from build123d import *

# Parameters (mm, degrees)
SKETCH1_R           = 7.5
SKETCH1_R_2         = 15
SKETCH1_R_3         = 11
SKETCH1_R_4         = 5
BOSS_EXTRUDE1_DEPTH = 10
SKETCH1_5_R         = 7.5
SKETCH1_5_R_2       = 5
BOSS_EXTRUDE2_DEPTH = 40
SKETCH2_R           = 7.5
SKETCH2_R_2         = 15
BOSS_EXTRUDE5_DEPTH = 10
SKETCH2_6_R         = 7.5
SKETCH2_6_R_2       = 5
BOSS_EXTRUDE6_DEPTH = 15
SKETCH2_7_R         = 15
SKETCH2_7_R_2       = 11
BOSS_EXTRUDE7_DEPTH = 30


with BuildPart() as part:
    # Sketch1 → Boss-Extrude1 (new body)
    # profile 1 of 6: a face of its own
    with BuildSketch(Plane(origin=(0, 0, 0), x_dir=(1, 0, 0), z_dir=(0, 1, 0))):
        with BuildLine():
            Line((-25, 35), (25, 35))
            ThreePointArc((25, 35), (32.071067812, 32.071067812), (35, 25))
            Line((35, 25), (35, -25))
            ThreePointArc((35, -25), (32.071067812, -32.071067812), (25, -35))
            Line((25, -35), (-25, -35))
            ThreePointArc((-25, -35), (-32.071067812, -32.071067812), (-35, -25))
            Line((-35, -25), (-35, 25))
            ThreePointArc((-35, 25), (-32.071067812, 32.071067812), (-25, 35))
        make_face()
        with Locations((25, -25)):
            Circle(SKETCH1_R, mode=Mode.SUBTRACT)
        Circle(SKETCH1_R_2, mode=Mode.SUBTRACT)
        with Locations((-25, 25)):
            Circle(SKETCH1_R, mode=Mode.SUBTRACT)
        with Locations((25, 25)):
            Circle(SKETCH1_R, mode=Mode.SUBTRACT)
        with Locations((-25, -25)):
            Circle(SKETCH1_R, mode=Mode.SUBTRACT)
    # profile 2 of 6: a face of its own
    with BuildSketch(Plane(origin=(0, 0, 0), x_dir=(1, 0, 0), z_dir=(0, 1, 0))):
        Circle(SKETCH1_R_2)
        with Locations(Location((0, 0, 0), (0, 0, 270))):
            Circle(SKETCH1_R_3, mode=Mode.SUBTRACT)
    # profile 3 of 6: a face of its own
    with BuildSketch(Plane(origin=(0, 0, 0), x_dir=(1, 0, 0), z_dir=(0, 1, 0))):
        with Locations((-25, -25)):
            Circle(SKETCH1_R)
        with Locations(Location((-25, -25, 0), (0, 0, 270))):
            Circle(SKETCH1_R_4, mode=Mode.SUBTRACT)
    # profile 4 of 6: a face of its own
    with BuildSketch(Plane(origin=(0, 0, 0), x_dir=(1, 0, 0), z_dir=(0, 1, 0))):
        with Locations((-25, 25)):
            Circle(SKETCH1_R)
        with Locations(Location((-25, 25, 0), (0, 0, 270))):
            Circle(SKETCH1_R_4, mode=Mode.SUBTRACT)
    # profile 5 of 6: a face of its own
    with BuildSketch(Plane(origin=(0, 0, 0), x_dir=(1, 0, 0), z_dir=(0, 1, 0))):
        with Locations((25, 25)):
            Circle(SKETCH1_R)
        with Locations(Location((25, 25, 0), (0, 0, 270))):
            Circle(SKETCH1_R_4, mode=Mode.SUBTRACT)
    # profile 6 of 6: a face of its own
    with BuildSketch(Plane(origin=(0, 0, 0), x_dir=(1, 0, 0), z_dir=(0, 1, 0))):
        with Locations((25, -25)):
            Circle(SKETCH1_R)
        with Locations(Location((25, -25, 0), (0, 0, 270))):
            Circle(SKETCH1_R_4, mode=Mode.SUBTRACT)
    extrude(amount=BOSS_EXTRUDE1_DEPTH)

    # Sketch1_5 → Boss-Extrude2 (add)
    # profile 1 of 4: a face of its own
    with BuildSketch(Plane(origin=(0, 0, 0), x_dir=(1, 0, 0), z_dir=(0, 1, 0))):
        with Locations(Location((-25, 25, 0), (0, 0, 270))):
            Circle(SKETCH1_5_R)
        with Locations(Location((-25, 25, 0), (0, 0, 270))):
            Circle(SKETCH1_5_R_2, mode=Mode.SUBTRACT)
    # profile 2 of 4: a face of its own
    with BuildSketch(Plane(origin=(0, 0, 0), x_dir=(1, 0, 0), z_dir=(0, 1, 0))):
        with Locations(Location((25, 25, 0), (0, 0, 270))):
            Circle(SKETCH1_5_R)
        with Locations(Location((25, 25, 0), (0, 0, 270))):
            Circle(SKETCH1_5_R_2, mode=Mode.SUBTRACT)
    # profile 3 of 4: a face of its own
    with BuildSketch(Plane(origin=(0, 0, 0), x_dir=(1, 0, 0), z_dir=(0, 1, 0))):
        with Locations(Location((-25, -25, 0), (0, 0, 270))):
            Circle(SKETCH1_5_R)
        with Locations(Location((-25, -25, 0), (0, 0, 270))):
            Circle(SKETCH1_5_R_2, mode=Mode.SUBTRACT)
    # profile 4 of 4: a face of its own
    with BuildSketch(Plane(origin=(0, 0, 0), x_dir=(1, 0, 0), z_dir=(0, 1, 0))):
        with Locations(Location((25, -25, 0), (0, 0, 270))):
            Circle(SKETCH1_5_R)
        with Locations(Location((25, -25, 0), (0, 0, 270))):
            Circle(SKETCH1_5_R_2, mode=Mode.SUBTRACT)
    extrude(amount=BOSS_EXTRUDE2_DEPTH)



with BuildPart() as body_2:
    # Sketch2 → Boss-Extrude5 (new body)
    with BuildSketch(Plane(origin=(0, 40, 0), x_dir=(1, 0, 0), z_dir=(0, 1, 0))):
        with BuildLine():
            ThreePointArc((35, 25), (32.071067812, 32.071067812), (25, 35))
            Line((25, 35), (-25, 35))
            ThreePointArc((-25, 35), (-32.071067812, 32.071067812), (-35, 25))
            Line((-35, 25), (-35, -25))
            ThreePointArc((-35, -25), (-32.071067812, -32.071067812), (-25, -35))
            Line((-25, -35), (25, -35))
            ThreePointArc((25, -35), (32.071067812, -32.071067812), (35, -25))
            Line((35, -25), (35, 25))
        make_face()
        with Locations(Location((-25, -25, 0), (0, 0, 270))):
            Circle(SKETCH2_R, mode=Mode.SUBTRACT)
        with Locations(Location((25, -25, 0), (0, 0, 270))):
            Circle(SKETCH2_R, mode=Mode.SUBTRACT)
        with Locations(Location((-25, 25, 0), (0, 0, 270))):
            Circle(SKETCH2_R, mode=Mode.SUBTRACT)
        with Locations(Location((0, 0, 0), (0, 0, 270))):
            Circle(SKETCH2_R_2, mode=Mode.SUBTRACT)
        with Locations(Location((25, 25, 0), (0, 0, 270))):
            Circle(SKETCH2_R, mode=Mode.SUBTRACT)
    extrude(amount=BOSS_EXTRUDE5_DEPTH)


with BuildPart() as part_1:
    add(part.part)

    add(body_2.part)  # Boss-Extrude6 merges body 2
    # Sketch2_6 → Boss-Extrude6 (add)
    # profile 1 of 4: a face of its own
    with BuildSketch(Plane(origin=(0, 40, 0), x_dir=(1, 0, 0), z_dir=(0, 1, 0))):
        with Locations(Location((25, 25, 0), (0, 0, 270))):
            Circle(SKETCH2_6_R)
        with Locations(Location((25, 25, 0), (0, 0, 270))):
            Circle(SKETCH2_6_R_2, mode=Mode.SUBTRACT)
    # profile 2 of 4: a face of its own
    with BuildSketch(Plane(origin=(0, 40, 0), x_dir=(1, 0, 0), z_dir=(0, 1, 0))):
        with Locations(Location((25, -25, 0), (0, 0, 270))):
            Circle(SKETCH2_6_R)
        with Locations(Location((25, -25, 0), (0, 0, 270))):
            Circle(SKETCH2_6_R_2, mode=Mode.SUBTRACT)
    # profile 3 of 4: a face of its own
    with BuildSketch(Plane(origin=(0, 40, 0), x_dir=(1, 0, 0), z_dir=(0, 1, 0))):
        with Locations(Location((-25, -25, 0), (0, 0, 270))):
            Circle(SKETCH2_6_R)
        with Locations(Location((-25, -25, 0), (0, 0, 270))):
            Circle(SKETCH2_6_R_2, mode=Mode.SUBTRACT)
    # profile 4 of 4: a face of its own
    with BuildSketch(Plane(origin=(0, 40, 0), x_dir=(1, 0, 0), z_dir=(0, 1, 0))):
        with Locations(Location((-25, 25, 0), (0, 0, 270))):
            Circle(SKETCH2_6_R)
        with Locations(Location((-25, 25, 0), (0, 0, 270))):
            Circle(SKETCH2_6_R_2, mode=Mode.SUBTRACT)
    extrude(amount=BOSS_EXTRUDE6_DEPTH)

    # Sketch2_7 → Boss-Extrude7 (add)
    with BuildSketch(Plane(origin=(0, 40, 0), x_dir=(1, 0, 0), z_dir=(0, 1, 0))):
        with Locations(Location((0, 0, 0), (0, 0, 270))):
            Circle(SKETCH2_7_R)
        with Locations(Location((0, 0, 0), (0, 0, 270))):
            Circle(SKETCH2_7_R_2, mode=Mode.SUBTRACT)
    extrude(amount=BOSS_EXTRUDE7_DEPTH)


solid = part_1.part
CAD build for the part. Positions are in the model's coordinates, mm. A direction names the side the tool comes from. Round coordinates to 2 decimals unless told otherwise and drop trailing zeros. Write each loop counter-clockwise with the first axis right and the second up, starting at its lowest first coordinate (ties: lowest second). Pieces come first, ordered by that corner, then holes.
(1) 3-axis set-ups, long thin cutter, end or side, ignore diameter. For faces 5 (the face through (-19.9, 52.5, 19.5)), 6 (the face through (30.1, 24.8, 19.5)), 7 (the face through (-35, 5, 0)): which of +Z, -Z, +X, -X, +Y, -Y reach the whole face in a straight line?
(2) Drop a flat-ended pin along its axis: P1, Ø4.5, axis at x = 22, z = -25, coming from the +Y side. Give the stop position or say it passes through.
(3) Slice it at C-C, the plane x = 0. Write the cut outline in (y, z), and give its area (3 significant figures).
(4) Slice it at B-B, the plane z = -26. Count the separate pieces of the cut face and the enclosed holes in it, and give its area (3 significant figures).
(5) Mould opens along Y. For faces 1 (the face through (0, 50, -16)), 2 (the face through (-8, 0, -8)), 3 (the face through (31.99, 44.93, 32.15)), 4 (the face through (-19.9, 24.8, 19.5)) say: pulls with the +Y half, pulls with the -Y half, needs draft (parallel to the pull), parting line crosses it, or undercut.
(6) Probe line 1 along X through (y, z) = (18, 25); line 2 along X through (y, z) = (51.75, 0); line 3 along Y through (x, z) = (-2.5, 27). List the from-to ranges inside material, lowest first.
(7) Slice it at A-A, the plane y = 31. Write the cut outline in (x, z).
From the geometry:
1. face 5: +Y
1. face 6: none
1. face 7: +Z, -Z, -X, +Y, -Y
2. P1: stops at y = 55
3. outline: (0, -35) - (10, -35) - (10, -11) - (0, -11) - close; (0, 11) - (10, 11) - (10, 35) - (0, 35) - close; (40, -35) - (50, -35) - (50, -15) - (70, -15) - (70, -11) - (40, -11) - close; (40, 11) - (70, 11) - (70, 15) - (50, 15) - (50, 35) - (40, 35) - close
3. area: 1,120 mm2
4. separate pieces: 3
4. enclosed holes: 1
4. area: 1,360 mm2
5. face 1: pulls with the +Y half
5. face 2: pulls with the -Y half
5. face 3: needs draft
5. face 4: undercut
6. line 1: x = -32.5 to -30, -20 to -17.5, 17.5 to 20, 30 to 32.5
6. line 2: x = -15 to -11, 11 to 15
6. line 3: y = 0 to 10, 40 to 50
7. outline: circle Ø15 at (-25, -25); circle Ø15 at (-25, 25); circle Ø15 at (25, -25); circle Ø15 at (25, 25); hole circle Ø10 at (-25, -25); hole circle Ø10 at (-25, 25); hole circle Ø10 at (25, -25); hole circle Ø10 at (25, 25)
